For this review, take the finished solid that the model builds, in its own axes (mm). Face numbers are marked on the shaded views. A direction names the side the tool comes from. Give positions to 0.01 mm unless a question says otherwise; leave off trailing zeros. Answer as CSV lines item,"result". Start each with the question number.
Item 1: For L1, parallel to Y at x = 0, z = 4; L2, parallel to Y at x = 0, z = 9.05, list the stretches that pass through material, from the lowest coordinate up. Write a range as from..to.
Item 2: Machinability: for the marked faces 4, 5 and 6, which of the approach directions +Z, -Z, +X, -X, +Y, -Y give a long, thin tool a straight path to every point of the face, cutting with its end or side? Answer none if there is none.
Item 3: Clearance check with flat-ended pins moving along their axes: P1, Ø4, axis at x = 6, z = 4, coming from the -Y side; P2, Ø1.5, axis at x = -6, z = 5, coming from the +Y side; P3, Ø5.5, axis at x = 0, y = 0, coming from the +Z side; P4, Ø2, axis at y = 2, z = 9.5, coming from the -X side. State where each tip first meets the part, or that it passes through.
Item 4: The part is to be moulded in two halves that separate along Y. For the marked faces 1, 2 and 3, say which applies: +Y half, -Y half, draft (parallel to the pull), parting line (faces both ways), or undercut.
```python
from build123d import *

# Parameters (mm, degrees)
F2_R = 0.3


with BuildPart() as f1:
    # F0 (on Front) → F1 (revolve)
    with BuildSketch(Plane.XZ):
        Polygon((-6, 0), (-3.5, 0), (-3.5, 8.000001), (-4.4, 8.000001), (-4.4, 12), (-12.4, 12), (-12.4, 11), (-13, 11), (-13, 10), (-12.4, 10), (-12.4, 7), (-7.203946, 7), (-6, 5.550987), align=None)
    revolve(axis=Axis((0, 0, 7.469198), (0, 0, 1)))

    # F2
    f2_edges = [f1.edges().sort_by_distance(p)[0] for p in [
        (12.4, 0, 12),
        (12.4, 0, 7),
        (6, 0, 0),
    ]]
    fillet(f2_edges, radius=F2_R)


solid = f1.part
```
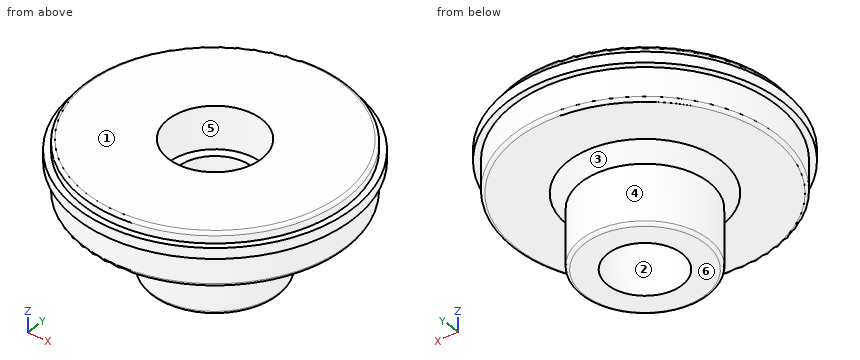
Computed values:
1,L1,"-6..-3.5, 3.5..6"
1,L2,"-12.4..-4.4, 4.4..12.4"
2,face 4,"-Z"
2,face 5,"+Z"
2,face 6,"-Z, +X, -X, +Y, -Y"
3,P1,"y = -4.47"
3,P2,"y = 2.9"
3,P3,"through"
3,P4,"x = -12.95"
4,face 1,"draft"
4,face 2,"undercut"
4,face 3,"parting line"
